Read the model definition and answer for the solid it produces. Units are mm, in the model's axes. A direction names the side the tool comes from. Round coordinates to 2 decimals unless told otherwise and drop trailing zeros. Order: outer loops, then holes, each group sorted by start corner. A loop starts at its lowest first (then second) coordinate and runs counter-clockwise, first axis right, second up. Notation, with made-up numbers: (20, 69) - (53, 69) arc R26 cw to (53, 94) - close; hole circle Ø8 at (-16, 10). An arc over 180 degrees is marked (long way). Answer as a JSON object with one key per item and string values. Group by question number.
Q1. A cutting plane is placed at B-B on y = 26. Determine the outline of the cut face in (x, z), and give its area (3 significant figures).
Q2. A cutting plane is placed at C-C on y = 9.5. Determine the outline of the cut face in (x, z) (3 decimals).
Q3. A tool of negligible diameter and unlimited length cuts with its end or side. For faces 5 (the flat face through (0.968, 36.325, -6.001)), 6 (the cylindrical face through (0.29, 16.66, -2.23)), from which of +Z, -Z, +X, -X, +Y, -Y can it reach the whole face along a straight path? Write none if from no direction.
Q4. Consider line 1 (X direction, y = 24.4, z = 0); line 2 (Z direction, x = 7.5, y = 24.5); line 3 (Z direction, x = 0, y = 24.35). Determine where each line is inside the solid, lowest interval first.
Q5. The mould has two halves that part along X. Classify faces 1 (the flat face through (5, 25, 0)), 2 (the cylindrical face through (9.169, 24.26, -0.526)), 3 (the flat face through (10, 24, 0)), 4 (the conical face through (-1.92, 5.07, 0.6)): pulls with the +X half, pulls with the -X half, needs draft (parallel to the pull), parting line crosses it, or undercut.
Q6. Given pin 1 Ø4.5 at (x, z) = (7.5, 0) entering from +Y; pin 2 Ø5 at (x, z) = (-3.5, 0) entering from +Y; pin 3 Ø6 at (x, z) = (3.5, -2.5) entering from +Y, each flat-ended and moving along its own axis, determine where each tip first touches the part or whether it passes through.
Q7. A cutting plane is placed at A-A on x = -7.5. Determine the outline of the cut face in (y, z).
Autodesk Inventor part; units mm, degrees
ref_plane "YZ Plane" through (0, 0, 0) normal (1, 0, 0) x (0, 1, 0)
ref_plane "XY Plane" through (0, 0, 0) normal (0, 0, 1) x (1, 0, 0)
sketch "Skizze1" plane through (0, 0, 0) normal (0, 0, 1) x (1, 0, 0)
  line L0 (-3.3, 0) -> (0.55, 0)
  line L1 (0, -6) -> (0, 36)
  line L2 (-1.25, 0) -> (-0.75, 0)
  line L3 (-0.75, 0) -> (-0.75, 30)
  line L4 (-0.75, 30) -> (-2.25, 30)
  line L5 (-2.25, 30) -> (-2.25, 10)
  line L6 (-2.25, 10) -> (-2.75, 10)
  line L7 (-2.75, 10) -> (-1.25, 0)
  point P0 (0, 0)
  dimension "d0" = 1.5
  dimension "d1" = 0.5
  dimension "d2" = 0.5
  dimension "d3" = 0.75
  dimension "d6" = 30
  dimension "d7" = 10
revolve "Umdrehung1" add sketch "Skizze1" angle 360 about axis through (0, -10, 0) along (0, 1, 0)
ref_plane "Arbeitsebene1" through (0, 50, 0) normal (0, 1, 0) x (-1, 0, 0)
sketch "Skizze3" plane through (0, 0, 0) normal (1, 0, 0) x (0, 1, 0)
  line L0 (30, -2.25) -> (30, 2.25)
  line L1 (30, 2.25) -> (26.6518, -2.25)
  line L2 (10, -2.25) -> (30, -2.25)
  line L3 (30, 2.25) -> (30, -2.25)
  line L4 (30, -2.25) -> (26.6518, -2.25)
  point P0 (0, 0)
extrude "Extrusion1" cut sketch "Skizze3" against normal mid plane 10
sketch "Skizze4" plane through (0, 28.3259, 0) normal (0, 0.8022892, -0.5969355) x (1, 0, 0)
  ellipse E0 centre (0, 0) end of major axis (0, -2.8045) minor radius 2.25
  ellipse E1 centre (0, 0) end of major axis (0, -2.8045) minor radius 2.25
  ellipse E2 centre (0, 0) end of major axis (0, -0.9255) minor radius 0.7538
  point P0 (0, 16.9087)
extrude "Extrusion2" add sketch "Skizze4" along normal blind 10
sketch "Skizze5" plane through (0, 0, 0) normal (1, 0, 0) x (0, 1, 0)
  line L0 (25, 2.25) -> (23.5, 2.25)
  line L1 (23.5, 2.25) -> (23.5, -2.25)
  line L2 (23.5, -2.25) -> (25, -2.25)
  line L3 (25, -2.25) -> (25, 2.25)
  line L4 (-7.6046, 0) -> (45.6275, 0)
  line L5 (0, -10.4132) -> (0, 4.9439)
  point P0 (0, 0)
  dimension "d23" = 4.5
  dimension "d24" = 2.25
  dimension "d25" = 25
  dimension "d26" = 1.5
extrude "Extrusion3" add sketch "Skizze5" along normal mid plane 20
sketch "Skizze6" plane through (0, 0, 0) normal (0, -1, 0) x (1, 0, 0)
  circle A0 centre (0, 0) radius 0.75
extrude "Extrusion4" cut sketch "Skizze6" against normal blind 27
sketch "Skizze7" plane through (0, 25, 2.25) normal (0, 1, 0) x (1, 0, 0)
  circle A0 centre (7.5, 2.25) radius 1.75
  circle A1 centre (-7.5, 2.25) radius 1.75
  line L0 (10, 4.5) -> (10, 0)
  point P0 (0, 2.25)
  dimension "d31" = 3.5
  dimension "d32" = 3.5
  dimension "d33" = 15
  dimension "d34" = 2.5
extrude "Extrusion5" cut sketch "Skizze7" against normal blind 5
properties part number "Düse"
Result set:
{
 "1": {"outline": "circle Ø4.5 at (0, 0); hole circle Ø1.5 at (0, 0)", "area": "14.1 mm²"},
 "2": {"outline": "circle Ø5.35 at (0, 0); hole circle Ø1.5 at (0, 0)"},
 "3": {"face 5": "-Z, +X, -X, +Y", "face 6": "none"},
 "4": {"line 1": "x = -10 to -9.25, -5.75 to -0.75, 0.75 to 5.75, 9.25 to 10", "line 2": "z = -2.25 to -1.75, 1.75 to 2.25", "line 3": "z = -2.25 to -0.75, 0.75 to 2.25"},
 "5": {"face 1": "needs draft", "face 2": "undercut", "face 3": "pulls with the +X half", "face 4": "parting line crosses it"},
 "6": {"pin 1": "stops at y = 25", "pin 2": "stops at y = 33.84", "pin 3": "stops at y = 37.9"},
 "7": {"outline": "(23.5, -2.25) - (25, -2.25) - (25, -1.75) - (23.5, -1.75) - close; (23.5, 1.75) - (25, 1.75) - (25, 2.25) - (23.5, 2.25) - close"}
}
